Work out the finished part from the listing and answer in its coordinate system (mm). Face numbers are marked on the shaded views. Coordinates: 2 decimals unless noted, no trailing zeros. Order: outer loops, then holes, each group sorted by start corner. A loop starts at its lowest first (then second) coordinate and runs counter-clockwise, first axis right, second up. Notation, with made-up numbers: (-19.5, -25) - (-4.5, -25) arc R23 cw to (-4.5, 13) - close; hole circle Ø8 at (33.25, 76). An arc over 180 degrees is marked (long way). Answer as a JSON object with one key per item and string values. Group by question number.
1) Section B-B (y = 9) is taken. Give the vertices of the cut face in (x, z).
2) Section A-A (x = 15.5) is taken. Give the vertices of the cut face in (y, z).
3) The mould has two halves that part along X. Classify the marked faces 1, 2, 3 and 4: released by +X, released by -X, zero draft, split by the parting line, or undercut.
4) Section C-C (z = -10) is taken. Give the vertices of the cut face in (x, y).
5) Section D-D (x = 0) is taken. Give the vertices of the cut face in (y, z), plus the area to 3 significant figures.
6) Find the intervals of material crossed by line 1 along Z through (x, y) = (-15.5, 7); line 2 along Z through (x, y) = (-15.5, 3.75); line 3 along X through (y, z) = (14, -30.5), in increasing order.
7) Each of these flat-tipped pins is pushed along its axis until it touches: P1, Ø1.2, axis at y = 2.5, z = -47.5, coming from the -X side; P2, Ø2, axis at x = 2, y = 2, coming from the -Z side; P3, Ø2, axis at x = 2, z = -46.5, coming from the -Y side. Where does it stop, or does it pass through?
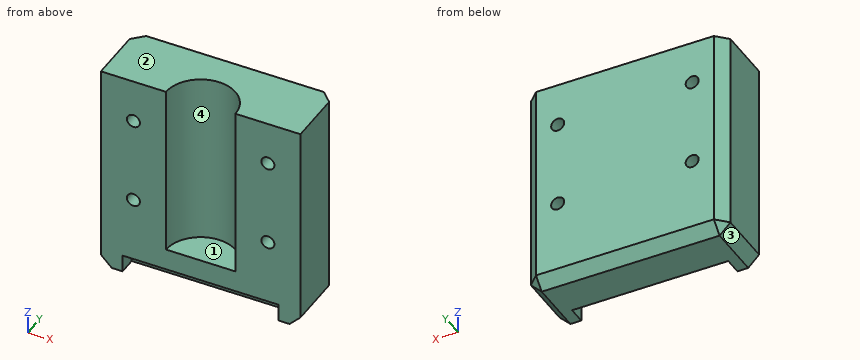
from build123d import *

# Parameters (mm, degrees)
Y_KSEKLIK_EKSTR_ZYON1_DEPTH = 45
IZIM2_W                     = 46
IZIM2_H                     = 5
Y_KSEKLIK_EKSTR_ZYON2_DEPTH = 14
Y_KSEKLIK_EKSTR_ZYON3_DEPTH = 4
PAH1_SIZE                   = 2.5
IZIM4_R                     = 1.5
KES_EKSTR_ZYON1_DEPTH       = 35


with BuildPart() as part:
    # Çizim1 → Yükseklik-Ekstrüzyon1 (new body)
    with BuildSketch(Plane.XY):
        with BuildLine():
            Line((-8, 0), (-23, 0))
            Line((-23, 0), (-23, 15))
            Line((-23, 15), (23, 15))
            Line((23, 15), (23, 0))
            Line((23, 0), (8, 0))
            ThreePointArc((8, 0), (0, 8), (-8, 0))
        make_face()
    extrude(amount=-Y_KSEKLIK_EKSTR_ZYON1_DEPTH)

    # Çizim2 → Yükseklik-Ekstrüzyon2 (add)
    with BuildSketch(Plane.XZ):
        with Locations((0, -42.5)):
            Rectangle(IZIM2_W, IZIM2_H)
    extrude(amount=-Y_KSEKLIK_EKSTR_ZYON2_DEPTH)

    # Çizim3 → Yükseklik-Ekstrüzyon3 (add)
    with BuildSketch(Plane(origin=(0, 0, -45), x_dir=(-1, 0, 0), z_dir=(0, 0, -1))):
        Polygon((-23, 15), (23, 15), (23, 4), (23, 0), (18, 0), (18, 4), (-18, 4), (-18, 0), (-23, 0), (-23, 4), align=None)
    extrude(amount=Y_KSEKLIK_EKSTR_ZYON3_DEPTH)

    # Pah1
    pah1_edges = [part.edges().sort_by_distance(p)[0] for p in [
        (-23, 15, -24.5),
        (23, 15, -24.5),
        (23, 7.5, -49),
        (-23, 7.5, -49),
        (0, 15, -49),
    ]]
    chamfer(pah1_edges, length=PAH1_SIZE)

    # Çizim4 → Kes-Ekstrüzyon1 (cut)
    with BuildSketch(Plane.XZ):
        with Locations((15.5, -10)):
            Circle(IZIM4_R)
        with Locations((15.5, -30)):
            Circle(IZIM4_R)
        with Locations(Location((-15.5, -30, 0), (0, 0, 180))):
            Circle(IZIM4_R)
        with Locations(Location((-15.5, -10, 0), (0, 0, 180))):
            Circle(IZIM4_R)
    extrude(amount=-KES_EKSTR_ZYON1_DEPTH, mode=Mode.SUBTRACT)


solid = part.part
Report:
{
 "1": {"outline": "(-23, -46.5) - (-20.5, -49) - (20.5, -49) - (23, -46.5) - (23, 0) - (-23, 0) - close; hole circle Ø3 at (-15.5, -30); hole circle Ø3 at (-15.5, -10); hole circle Ø3 at (15.5, -30); hole circle Ø3 at (15.5, -10)"},
 "2": {"outline": "(0, -45) - (4, -45) - (4, -49) - (12.5, -49) - (15, -46.5) - (15, -31.5) - (0, -31.5) - close; (0, -28.5) - (15, -28.5) - (15, -11.5) - (0, -11.5) - close; (0, -8.5) - (15, -8.5) - (15, 0) - (0, 0) - close"},
 "3": {"face 1": "undercut", "face 2": "zero draft", "face 3": "released by -X", "face 4": "undercut"},
 "4": {"outline": "(-23, 0) - (-17, 0) - (-17, 15) - (-20.5, 15) - (-23, 12.5) - close; (-14, 0) - (-8, 0) arc R8 cw to (8, 0) - (14, 0) - (14, 15) - (-14, 15) - close; (17, 0) - (23, 0) - (23, 12.5) - (20.5, 15) - (17, 15) - close"},
 "5": {"outline": "(0, -45) - (4, -45) - (4, -49) - (12.5, -49) - (15, -46.5) - (15, 0) - (8, 0) - (8, -40) - (0, -40) - close", "area": "396 mm²"},
 "6": {"line 1": "z = -49 to -31.5, -28.5 to -11.5, -8.5 to 0", "line 2": "z = -45 to -31.5, -28.5 to -11.5, -8.5 to 0", "line 3": "x = -21.5 to -16.91, -14.09 to 14.09, 16.91 to 21.5"},
 "7": {"P1": "stops at x = -22.6", "P2": "stops at z = -45", "P3": "stops at y = 4"}
}
